Autodesk Inventor part; units mm, degrees
ref_plane "YZ Plane" through (0, 0, 0) normal (1, 0, 0) x (0, 1, 0)
ref_plane "XZ Plane" through (0, 0, 0) normal (0, 1, 0) x (-1, 0, 0)
ref_plane "XY Plane" through (0, 0, 0) normal (0, 0, 1) x (1, 0, 0)
sketch "Szkic1" plane through (0, 0, 0) normal (0, 1, 0) x (-1, 0, 0)
  circle A0 centre (0, 0) radius 26.738
  dimension "d0" = 26.738
extrude "Wyciągnięcie proste1" add sketch "Szkic1" along normal blind 5
sketch "Szkic2" plane through (0, 5, 0) normal (0, 1, 0) x (1, 0, 0)
  circle A0 centre (-1.4324, 0) radius 18.869 construction
  circle A1 centre (-20.3014, 0) radius 3.4345
  point P0 (0, 0)
  dimension "d5" = 3.4345
  dimension "d6" = 18.869
extrude "Wyciągnięcie proste2" add sketch "Szkic2" along normal blind 6
pattern_circular "Szyk kołowy1" count 6 over 360 about axis through (0, 0, 0) along (0, 1, 0) of "Wyciągnięcie proste2"
sketch "Szkic5" plane through (0, 0, 0) normal (0, -1, 0) x (1, 0, 0)
  point P0 (0, 0)
sketch "Szkic6" plane through (0, 0, 0) normal (0, -1, 0) x (1, 0, 0)
  circle A0 centre (0, 0) radius 13.2
  dimension "d17" = 13.2
extrude "Wyciągnięcie proste5" add sketch "Szkic6" along normal blind 12
sketch "Szkic7" plane through (0, 5, 0) normal (0, 1, 0) x (1, 0, 0)
  circle A0 centre (0, 0) radius 11
  dimension "d20" = 11
extrude "Wyciągnięcie proste6" cut sketch "Szkic7" against normal blind 6
equation "\"d0\" = R"
equation "\"d3\" = h2"
equation "\"d5\" = dwr1"
equation "\"d17\" = 1.2 * Lrz"
equation "\"d18\" = h2 + Lh"
equation "\"d20\" = Lrz"
equation "\"silnik_rw\" = 2.5"
equation "\"silnik_d_srub\" = 31"
equation "\"silnik_r_wypust\" = Lrz"
equation "\"Lrz\" = 11"
equation "\"Lh\" = 7"
equation "\"Lrw\" = 4"
equation "\"h2\" = 5"
equation "\"h1\" = 2"
equation "\"Rr\" = 2"
equation "\"E1\" = 1"
equation "\"dwr\" = R"
equation "\"dwr2\" = 0.5 * Lrz + 0.5 * R"
equation "\"dwr1\" = -0.25 * Rr + 0.25 * R - 0.25 * Lrz"
equation "\"R1\" = 5"
equation "\"korpus_rw\" = 36.5"
properties part number "Dysk_wy"
Design review of the part built by this model. Coordinates are the model's own, in mm. A direction names the side the tool comes from. Give positions to 0.01 mm unless a question says otherwise; leave off trailing zeros. Order: outer loops, then holes, each group sorted by start corner. A loop starts at its lowest first (then second) coordinate and runs counter-clockwise, first axis right, second up.
1. Add section C-C, the plane y = 5.75. State the section outline as (x, z) points, then the cut area to 3 significant figures.
Solution:
outline: circle Ø6.87 at (-20.3, 0); circle Ø6.87 at (-10.15, -17.58); circle Ø6.87 at (-10.15, 17.58); circle Ø6.87 at (10.15, -17.58); circle Ø6.87 at (10.15, 17.58); circle Ø6.87 at (20.3, 0)
area: 222 mm2
2. Tool access review of faces 1 (the flat face through (0, 5, -12)), 2 (the flat face through (-6, 0, 12)), 3 (the flat face through (10, 11, -18)): name each direction out of +Z, -Z, +X, -X, +Y, -Y from which nothing blocks a thin tool from reaching the whole face with its end or side.
Solution:
face 1: +Y
face 2: -Y
face 3: +Z, -Z, +X, -X, +Y
3. For pin 1 Ø6.5 at (x, z) = (0.5, -2) entering from +Y; pin 2 Ø4 at (x, y) = (-9.5, -8.5) entering from +Z; pin 3 Ø8 at (x, z) = (14, -21) entering from -Y, all flat-tipped, find the tip position at first contact; note any pin that passes through.
Solution:
pin 1: stops at y = -1
pin 2: stops at z = 10.86
pin 3: stops at y = 0
4. Add section B-B, the plane x = -22. State the section outline as (y, z) points, then the cut area to 3 significant figures.
Solution:
outline: (0, -15.2) - (5, -15.2) - (5, -2.99) - (11, -2.99) - (11, 2.99) - (5, 2.99) - (5, 15.2) - (0, 15.2) - close
area: 188 mm2
5. Mouldability with a two-part tool opening along Z and no side actions: class faces 4 (the flat face through (20, 11, 0)), 5 (the cylindrical face through (-13.427, 7.958, -18.613)), 6 (the cylindrical face through (-23.733, 7.958, 0.151)) as +Z half, -Z half, draft (parallel to the pull), parting line (faces both ways), or undercut.
Solution:
face 4: draft
face 5: undercut
face 6: parting line
6. Add section A-A, the plane z = 0. State the section outline as (x, y) points, then the cut area to 3 significant figures.
Solution:
outline: (-26.74, 0) - (-13.2, 0) - (-13.2, -12) - (13.2, -12) - (13.2, 0) - (26.74, 0) - (26.74, 5) - (23.74, 5) - (23.74, 11) - (16.87, 11) - (16.87, 5) - (11, 5) - (11, -1) - (-11, -1) - (-11, 5) - (-16.87, 5) - (-16.87, 11) - (-23.74, 11) - (-23.74, 5) - (-26.74, 5) - close
area: 535 mm2
7. To check wall thickness, follow L1, parallel to Z at x = 0, y = 2.8; L2, parallel to Y at x = 4, z = 4.5; L3, parallel to Y at x = -24, z = -2.5. State the ranges of each line that lie inside material, in increasing order.
Solution:
L1: z = -26.74 to -11, 11 to 26.74
L2: y = -12 to -1
L3: y = 0 to 5
8. Add section D-D, the plane y = 2.75. State the section outline as (x, z) points.
Solution:
outline: circle Ø53.48 at (0, 0); hole circle Ø22 at (0, 0)
